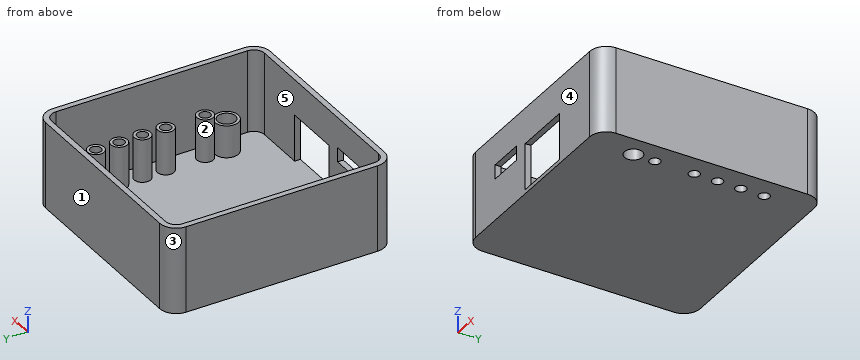
from build123d import *

# Parameters (mm, degrees)
PARED_DEPTH             = 23
CONECTORES_REACH        = 92.181
CROQUIS2_W              = 16
CROQUIS2_H              = 13
CROQUIS2_W_2            = 10
CROQUIS2_H_2            = 4
BASE_START              = -1.12
BASE_FRENTE_DEPTH       = 1.12
LUCES_REACH             = 91.076
CROQUIS3_R              = 1.5
CROQUIS3_R_2            = 2.5
SALIENTE_EXTRUIR1_START = 12
CROQUIS3_3_R            = 2.3
CROQUIS3_3_R_2          = 1.5
SALIENTE_EXTRUIR1_DEPTH = 12
SALIENTE_EXTRUIR2_START = 9
CROQUIS3_4_R            = 3.3
CROQUIS3_4_R_2          = 2.5
SALIENTE_EXTRUIR2_DEPTH = 9


with BuildPart() as part:
    # Croquis1 → pared (new body)
    with BuildSketch(Plane.XY):
        with BuildLine():
            Line((3, 61.1), (56, 61.1))
            ThreePointArc((56, 61.1), (59.252691193, 59.752691193), (60.6, 56.5))
            Line((60.6, 56.5), (60.6, 3))
            ThreePointArc((60.6, 3), (59.252691193, -0.252691193), (56, -1.6))
            Line((56, -1.6), (3, -1.6))
            ThreePointArc((3, -1.6), (-0.252691193, -0.252691193), (-1.6, 3))
            Line((-1.6, 3), (-1.6, 56.5))
            ThreePointArc((-1.6, 56.5), (-0.252691193, 59.752691193), (3, 61.1))
        make_face()
        with BuildLine():
            Line((3, 0), (56, 0))
            ThreePointArc((56, 0), (58.121320344, 0.878679656), (59, 3))
            Line((59, 3), (59, 56.5))
            ThreePointArc((59, 56.5), (58.121320344, 58.621320344), (56, 59.5))
            Line((56, 59.5), (3, 59.5))
            ThreePointArc((3, 59.5), (0.878679656, 58.621320344), (0, 56.5))
            Line((0, 56.5), (0, 3))
            ThreePointArc((0, 3), (0.878679656, 0.878679656), (3, 0))
        make_face(mode=Mode.SUBTRACT)
    extrude(amount=PARED_DEPTH)

    # Croquis2 → conectores (cut, up to next)
    with BuildSketch(Plane.XZ.offset(1.6), mode=Mode.PRIVATE) as conectores_sk1:
        with Locations((34, 6.5)):
            Rectangle(CROQUIS2_W, CROQUIS2_H)
    conectores_tool1 = extrude(conectores_sk1.sketch, amount=-CONECTORES_REACH, mode=Mode.PRIVATE) & part.part
    # Croquis2 → conectores (cut, up to next)
    with BuildSketch(Plane.XZ.offset(1.6), mode=Mode.PRIVATE) as conectores_sk2:
        with Locations((17, 12.5)):
            Rectangle(CROQUIS2_W_2, CROQUIS2_H_2)
    conectores_tool2 = extrude(conectores_sk2.sketch, amount=-CONECTORES_REACH, mode=Mode.PRIVATE) & part.part
    add(conectores_tool1.solids().sort_by_distance((34, -1.6, 6.5))[0], mode=Mode.SUBTRACT)
    add(conectores_tool2.solids().sort_by_distance((17, -1.6, 12.5))[0], mode=Mode.SUBTRACT)

    # Croquis1<2> → base frente (add)
    with BuildSketch(Plane.XY.offset(BASE_START)):
        with BuildLine():
            Line((3, 61.1), (56, 61.1))
            ThreePointArc((56, 61.1), (59.252691193, 59.752691193), (60.6, 56.5))
            Line((60.6, 56.5), (60.6, 3))
            ThreePointArc((60.6, 3), (59.252691193, -0.252691193), (56, -1.6))
            Line((56, -1.6), (3, -1.6))
            ThreePointArc((3, -1.6), (-0.252691193, -0.252691193), (-1.6, 3))
            Line((-1.6, 3), (-1.6, 56.5))
            ThreePointArc((-1.6, 56.5), (-0.252691193, 59.752691193), (3, 61.1))
        make_face()
    extrude(amount=BASE_FRENTE_DEPTH)

    # Croquis3 → luces (cut, up to next)
    with BuildSketch(Plane.XY, mode=Mode.PRIVATE) as luces_sk1:
        with Locations((54.5, 48)):
            Circle(CROQUIS3_R)
    luces_tool1 = extrude(luces_sk1.sketch, amount=-LUCES_REACH, mode=Mode.PRIVATE) & part.part
    # Croquis3 → luces (cut, up to next)
    with BuildSketch(Plane.XY, mode=Mode.PRIVATE) as luces_sk2:
        with Locations((54.5, 41.5)):
            Circle(CROQUIS3_R)
    luces_tool2 = extrude(luces_sk2.sketch, amount=-LUCES_REACH, mode=Mode.PRIVATE) & part.part
    # Croquis3 → luces (cut, up to next)
    with BuildSketch(Plane.XY, mode=Mode.PRIVATE) as luces_sk3:
        with Locations((54.5, 35)):
            Circle(CROQUIS3_R)
    luces_tool3 = extrude(luces_sk3.sketch, amount=-LUCES_REACH, mode=Mode.PRIVATE) & part.part
    # Croquis3 → luces (cut, up to next)
    with BuildSketch(Plane.XY, mode=Mode.PRIVATE) as luces_sk4:
        with Locations((54.5, 28.5)):
            Circle(CROQUIS3_R)
    luces_tool4 = extrude(luces_sk4.sketch, amount=-LUCES_REACH, mode=Mode.PRIVATE) & part.part
    # Croquis3 → luces (cut, up to next)
    with BuildSketch(Plane.XY, mode=Mode.PRIVATE) as luces_sk5:
        with Locations((54.5, 17.5)):
            Circle(CROQUIS3_R)
    luces_tool5 = extrude(luces_sk5.sketch, amount=-LUCES_REACH, mode=Mode.PRIVATE) & part.part
    # Croquis3 → luces (cut, up to next)
    with BuildSketch(Plane.XY, mode=Mode.PRIVATE) as luces_sk6:
        with Locations((54.5, 11.5)):
            Circle(CROQUIS3_R_2)
    luces_tool6 = extrude(luces_sk6.sketch, amount=-LUCES_REACH, mode=Mode.PRIVATE) & part.part
    add(luces_tool1.solids().sort_by_distance((54.5, 48, 0))[0], mode=Mode.SUBTRACT)
    add(luces_tool2.solids().sort_by_distance((54.5, 41.5, 0))[0], mode=Mode.SUBTRACT)
    add(luces_tool3.solids().sort_by_distance((54.5, 35, 0))[0], mode=Mode.SUBTRACT)
    add(luces_tool4.solids().sort_by_distance((54.5, 28.5, 0))[0], mode=Mode.SUBTRACT)
    add(luces_tool5.solids().sort_by_distance((54.5, 17.5, 0))[0], mode=Mode.SUBTRACT)
    add(luces_tool6.solids().sort_by_distance((54.5, 11.5, 0))[0], mode=Mode.SUBTRACT)

    # Croquis3<3> → Saliente-Extruir1 (add)
    # profile 1 of 5: a face of its own
    with BuildSketch(Plane.XY.offset(SALIENTE_EXTRUIR1_START)):
        with Locations((54.5, 17.5)):
            Circle(CROQUIS3_3_R)
        with Locations((54.5, 17.5)):
            Circle(CROQUIS3_3_R_2, mode=Mode.SUBTRACT)
    # profile 2 of 5: a face of its own
    with BuildSketch(Plane.XY.offset(SALIENTE_EXTRUIR1_START)):
        with Locations((54.5, 28.5)):
            Circle(CROQUIS3_3_R)
        with Locations((54.5, 28.5)):
            Circle(CROQUIS3_3_R_2, mode=Mode.SUBTRACT)
    # profile 3 of 5: a face of its own
    with BuildSketch(Plane.XY.offset(SALIENTE_EXTRUIR1_START)):
        with Locations((54.5, 35)):
            Circle(CROQUIS3_3_R)
        with Locations((54.5, 35)):
            Circle(CROQUIS3_3_R_2, mode=Mode.SUBTRACT)
    # profile 4 of 5: a face of its own
    with BuildSketch(Plane.XY.offset(SALIENTE_EXTRUIR1_START)):
        with Locations((54.5, 41.5)):
            Circle(CROQUIS3_3_R)
        with Locations((54.5, 41.5)):
            Circle(CROQUIS3_3_R_2, mode=Mode.SUBTRACT)
    # profile 5 of 5: a face of its own
    with BuildSketch(Plane.XY.offset(SALIENTE_EXTRUIR1_START)):
        with Locations((54.5, 48)):
            Circle(CROQUIS3_3_R)
        with Locations((54.5, 48)):
            Circle(CROQUIS3_3_R_2, mode=Mode.SUBTRACT)
    extrude(amount=-SALIENTE_EXTRUIR1_DEPTH)

    # Croquis3<4> → Saliente-Extruir2 (add)
    with BuildSketch(Plane.XY.offset(SALIENTE_EXTRUIR2_START)):
        with Locations((54.5, 11.5)):
            Circle(CROQUIS3_4_R)
        with Locations((54.5, 11.5)):
            Circle(CROQUIS3_4_R_2, mode=Mode.SUBTRACT)
    extrude(amount=-SALIENTE_EXTRUIR2_DEPTH)


solid = part.part
Check sheet for the modelled part. Datum: model origin and axes. Units: mm. Face numbers are marked on the shaded views. A direction names the side the tool comes from. Give positions to 0.01 mm unless a question says otherwise; leave off trailing zeros. Write each loop counter-clockwise with the first axis right and the second up, starting at its lowest first coordinate (ties: lowest second). Pieces come first, ordered by that corner, then holes. Notation, with made-up numbers: M 0,-5 L 16,-5 A15 cw 16,8 Z; hole C 58.5,-20 d10. An arc over 180 degrees is marked long. Use one line per item in the form item = value.
(1) Tool access check on the marked faces 4 and 5. Record the directions out of +Z, -Z, +X, -X, +Y, -Y that give a thin tool (end or side, any length) a straight path to the whole face; none if there is none.
Answer block:
face_4 = +Z, -Z, +X, -X, -Y
face_5 = +Z
(2) Section check C-C on x = 38.5. Record the boundary of the cut face in (y, z).
Answer block:
outline = M -1.6,-1.12 L 61.1,-1.12 L 61.1,23 L 59.5,23 L 59.5,0 L -1.6,0 Z; M -1.6,13 L 0,13 L 0,23 L -1.6,23 Z
(3) Material ranges on line 1 along X through (y, z) = (38.5, 15.5); line 2 along Y through (x, z) = (41, 14.75); line 3 along X through (y, z) = (50, 11.5), recorded low to high.
Answer block:
line_1 = -1.6 to 0, 59 to 60.6
line_2 = -1.6 to 0, 59.5 to 61.1
line_3 = -1.6 to 0, 53.36 to 55.64, 59 to 60.6
(4) Draft check along X on the marked faces 1, 2 and 3. Enter one of: pulls with the +X half, pulls with the -X half, needs draft (parallel to the pull), parting line crosses it, or undercut.
Answer block:
face_1 = needs draft
face_2 = undercut
face_3 = pulls with the -X half
(5) Depth check by flat-ended pin: P1, Ø6, axis at x = 40.5, z = 3.5, coming from the -Y side; P2, Ø2.5, axis at x = 55.5, y = 35.5, coming from the +Z side; P3, Ø0.8, axis at y = -0.5, z = 12.5, coming from the -X side; P4, Ø5.5, axis at x = 54.5, y = 10.5, coming from the +Z side. Enter the tip coordinate at first touch or a pass-through.
Answer block:
P1 = -1.6
P2 = 12
P3 = -0.4
P4 = 9
(6) Section check B-B on z = 3. State how many separate pieces and enclosed holes the cut face has, plus the area to 3 significant figures.
Answer block:
separate_pieces = 7
enclosed_holes = 6
area = 416 mm2
(7) Section check A-A on y = 35. Record the boundary of the cut face in (x, z), plus the area to 3 significant figures.
Answer block:
outline = M -1.6,-1.12 L 53,-1.12 L 53,12 L 52.2,12 L 52.2,0 L 0,0 L 0,23 L -1.6,23 Z; M 56,-1.12 L 60.6,-1.12 L 60.6,23 L 59,23 L 59,0 L 56.8,0 L 56.8,12 L 56,12 Z
area = 159 mm2
